The listing builds one solid part. Answer for the finished solid, in the listing's coordinates (mm). A direction names the side the tool comes from. Give positions to 0.01 mm unless a question says otherwise; leave off trailing zeros. Order: outer loops, then holes, each group sorted by start corner. A loop starts at its lowest first (then second) coordinate and runs counter-clockwise, first axis right, second up. Notation, with made-up numbers: (-20, -38.75) - (-5, -38.75) arc R20 cw to (-5, -1.75) - close; hole circle Ø4 at (46, -2.5). An arc over 180 degrees is marked (long way). Use a Markdown table: item, result. Add a question column.
1) The mould has two halves that part along X. Classify faces 4 (the face through (-4.75, 0.89, -4.19)), 5 (the face through (3.5, 1, 1)), 6 (the face through (6.5, 1, -3)): released by +X, released by -X, zero draft, split by the parting line, or undercut.
2) Straight lines are drawn through the part: line 1 (X direction, y = 0.3, z = 1.5); line 2 (Z direction, x = 2.25, y = 0.2); line 3 (X direction, y = 0.1, z = -2.5). For each, find the intervals that lie inside material, in ascending order.
3) Find section A-A, the plane z = 0.75. Determine the outline of the cut face in (x, y).
4) Find section D-D, the plane z = -7. Determine the outline of the cut face in (x, y).
5) For faces 1 (the face through (-6.5, 1, -1)), 2 (the face through (-2.206, 0.887, -4.473)), 3 (the face through (-3.5, 1, 1)), determine the directions among +Z, -Z, +X, -X, +Y, -Y from which every point of the face is accessible in a straight line to the end or side of a thin tool.
6) A flat-ended cylindrical pin translates along its axis: pin 1 (6 mm diameter, centred on x = -0.5, z = -4.5, fed in from -Y). Find the tip coordinate at first contact, or state that the pin passes through.
7) Find section B-B, the plane x = 2. Determine the outline of the cut face in (y, z).
from build123d import *

# Parameters (mm, degrees)
BOSS_EXTRUDE1_DEPTH = 1.8
FILLET1_R           = 2
FILLET3_R           = 1


# Some blends are built 0.0001 mm under size
with BuildPart() as part:
    # Sketch1 → Boss-Extrude1 (new body)
    with BuildSketch(Plane(origin=(0, 0, 0), x_dir=(1, 0, 0), z_dir=(0, 1, 0))):
        with BuildLine():
            Line((6.5, 2.5), (6.5, 0))
            Line((6.5, 0), (6.5, -2))
            Line((6.5, -2), (3.5, -2))
            Line((3.5, -2), (3.5, 0))
            Line((3.5, 0), (-3.5, 0))
            Line((-3.5, 0), (-3.5, -2))
            Line((-3.5, -2), (-6.5, -2))
            Line((-6.5, -2), (-6.5, 0))
            Line((-6.5, 0), (-6.5, 2.5))
            Line((-6.5, 2.5), (-6.5, 3.5))
            Line((-6.5, 3.5), (-2.95, 4.9))
            Line((-2.95, 4.9), (-1.95, 4.9))
            ThreePointArc((-1.95, 4.9), (0.286343304, 2.198397365), (3.358114035, 3.890766339))
            ThreePointArc((3.358114035, 3.890766339), (3.298735092, 6.048400165), (1.7, 7.498557292))
            Line((1.7, 7.498557292), (1.7, 8.498557292))
            Line((1.7, 8.498557292), (6.5, 8.498557292))
            Line((6.5, 8.498557292), (6.5, 4.9))
            Line((6.5, 4.9), (6.5, 2.5))
        make_face()
    extrude(amount=BOSS_EXTRUDE1_DEPTH)

    # Fillet1
    # the kernel refuses this fillet: 2 mm, written as the material it takes off along each edge
    with BuildSketch(Plane(origin=(-1.95, -2.821440468, -4.9), x_dir=(0.20519567041703063, 0, 0.9787209698591859), z_dir=(0, 1, 0))) as fillet1_piece_1:
        with BuildLine():
            CenterArc((1.538967528, -1.95744194), FILLET1_R, 101.840953646, 48.860489585)
            Line((-0.20519567, -0.97872097), (-0.240078934, -0.95914655))
            ThreePointArc((-0.240078934, -0.95914655), (-0.141746674, -0.481152658), (-0.039148839, 0.008207827))
            Line((-0.039148839, 0.008207827), (0.008207827, 0.039148839))
            ThreePointArc((0.008207827, 0.039148839), (0.564288094, -0.018517333), (1.12036836, 0.039148839))
            Line((1.12036836, 0.039148839), (1.128576187, 0))
        make_face()
    extrude(amount=7.442880936, mode=Mode.SUBTRACT)

    # Fillet3
    fillet3_edges = [part.edges().sort_by_distance(p)[0] for p in [
        (1.7, 0.9, -8.498557292),
    ]]
    fillet(fillet3_edges, radius=FILLET3_R - 0.0001)  # a hair under: the kernel refuses the full size


solid = part.part
The answers:
| question | item | result |
|---|---|---|
| 1 | face 4 | released by -X |
| 1 | face 5 | undercut |
| 1 | face 6 | released by +X |
| 2 | line 1 | -6.5 to -3.5, 3.5 to 6.5 |
| 2 | line 2 | -8.39 to -7.24, -2.56 to 0 |
| 2 | line 3 | -6.5 to -0.54, 2.14 to 6.5 |
| 3 | outline | (-6.5, 0) - (-3.5, 0) - (-3.5, 1.8) - (-6.5, 1.8) - close; (3.5, 0) - (6.5, 0) - (6.5, 1.8) - (3.5, 1.8) - close |
| 4 | outline | (2.58, 0) - (6.5, 0) - (6.5, 1.8) - (2.58, 1.8) - close |
| 5 | face 1 | +Z, -Z, -X, +Y, -Y |
| 5 | face 2 | -Z, +Y, -Y |
| 5 | face 3 | +Z, +Y, -Y |
| 6 | pin 1 | y = 0 |
| 7 | outline | (0, -8.21) - (1.8, -8.21) - (1.8, -7.37) - (0, -7.37) - close; (0, -2.43) - (1.8, -2.43) - (1.8, 0) - (0, 0) - close |
